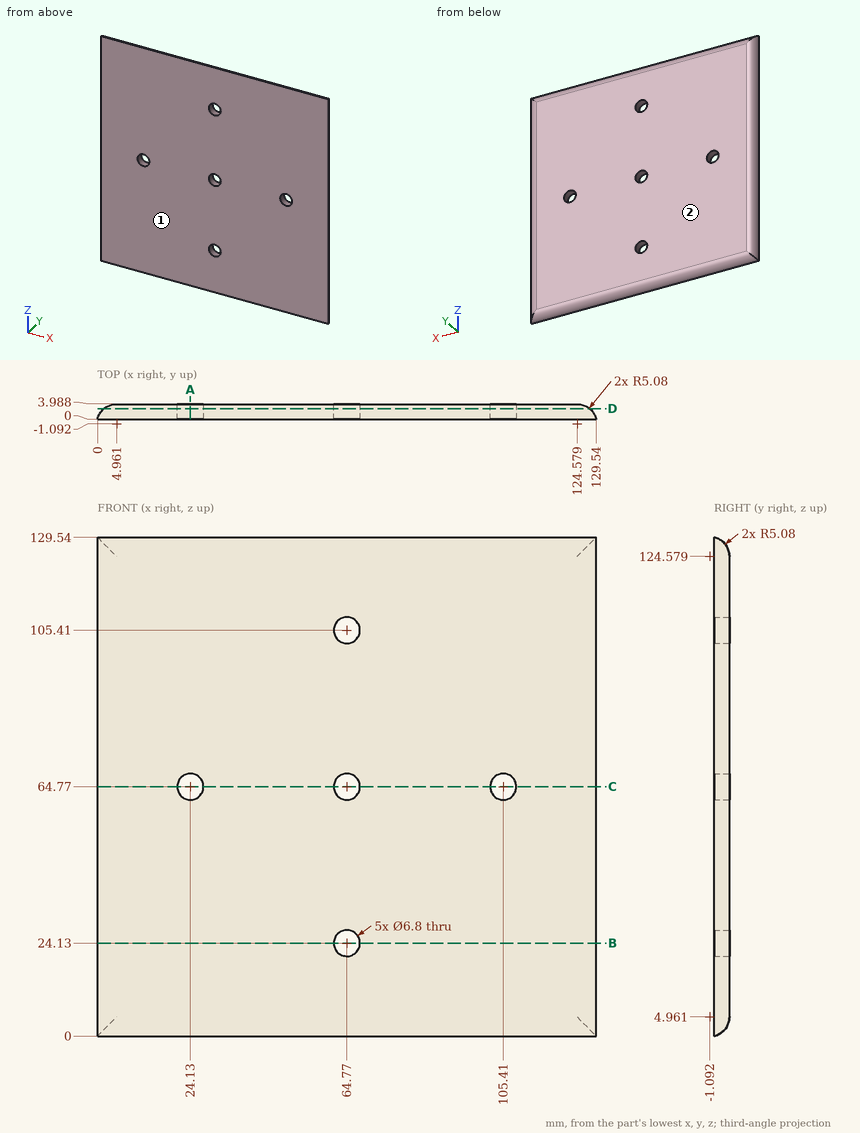
Geometry check sheet. Reference: drawing and pictorial views, mm from the part's lowest x, y, z. Round coordinates to 2 decimals unless told otherwise and drop trailing zeros. Write each loop counter-clockwise with the first axis right and the second up, starting at its lowest first coordinate (ties: lowest second). Pieces come first, ordered by that corner, then holes. Notation, with made-up numbers: (27.5, 27.25) -> (80.5, 27.25) arc R24 cw to (80.5, 41.25) -> close; hole circle Ø8 at (-30, 80.25). An arc over 180 degrees is marked (long way). Answer as CSV lines item,"result". Start each with the question number.
1) Go/stop test with flat-tipped pins: P1, Ø1.5, axis at y = 1, z = 70, coming from the -X side; P2, Ø2, axis at y = 1.5, z = 53, coming from the +X side. Record where each tip stops, or that it passes through.
2) Material ranges on line 1 (Z direction, x = 64.77, y = 2.4); line 2 (Z direction, x = 106.5, y = 1.15); line 3 (Z direction, x = 24.13, y = 2.35) (1 decimal), recorded low to high. Write a range as from..to.
3) Section check B-B on z = 24.13. Enter the section's corners in (x, y).
4) Section check C-C on z = 64.77. Enter the section's corners in (x, y), and give its area (3 significant figures).
5) Section check A-A on x = 24.13. Enter the section's corners in (y, z).
6) Release check for a two-part mould opening along Y. For the marked faces 1 and 2 record: pulls with the +Y half, pulls with the -Y half, needs draft (parallel to the pull), parting line crosses it, or undercut.
7) Section check D-D on y = 2.8. Enter the section's corners in (x, z).
Found:
1,P1,"stops at x = 0.06"
1,P2,"stops at x = 129.4"
2,line 1,"z = 1.27..20.73, 27.53..61.37, 68.17..102.01, 108.81..128.27"
2,line 2,"z = 0.4..61.55, 67.99..129.14"
2,line 3,"z = 1.2..61.4, 68.2..128.3"
3,outline,"(0, 0) -> (61.37, 0) -> (61.37, 3.99) -> (4.96, 3.99) arc R5.08 ccw to start; (68.17, 0) -> (129.54, 0) arc R5.08 ccw to (124.58, 3.99) -> (68.17, 3.99) -> close"
4,outline,"(0, 0) -> (20.73, 0) -> (20.73, 3.99) -> (4.96, 3.99) arc R5.08 ccw to start; (27.53, 0) -> (61.37, 0) -> (61.37, 3.99) -> (27.53, 3.99) -> close; (68.17, 0) -> (102.01, 0) -> (102.01, 3.99) -> (68.17, 3.99) -> close; (108.81, 0) -> (129.54, 0) arc R5.08 ccw to (124.58, 3.99) -> (108.81, 3.99) -> close"
4,area,"425 mm^2"
5,outline,"(0, 0) arc R5.08 ccw to (3.99, 4.96) -> (3.99, 61.37) -> (0, 61.37) -> close; (0, 68.17) -> (3.99, 68.17) -> (3.99, 124.58) arc R5.08 ccw to (0, 129.54) -> close"
6,face 1,"pulls with the -Y half"
6,face 2,"pulls with the +Y half"
7,outline,"(1.7, 1.7) -> (127.84, 1.7) -> (127.84, 127.84) -> (1.7, 127.84) -> close; hole circle Ø6.8 at (24.13, 64.77); hole circle Ø6.8 at (64.77, 24.13); hole circle Ø6.8 at (64.77, 64.77); hole circle Ø6.8 at (64.77, 105.41); hole circle Ø6.8 at (105.41, 64.77)"
